The model under review builds one solid part; all positions refer to its coordinate system, in mm. Face numbers are marked on the shaded views. A direction names the side the tool comes from. Coordinates: 2 decimals unless noted, no trailing zeros. Order: outer loops, then holes, each group sorted by start corner. A loop starts at its lowest first (then second) coordinate and runs counter-clockwise, first axis right, second up.
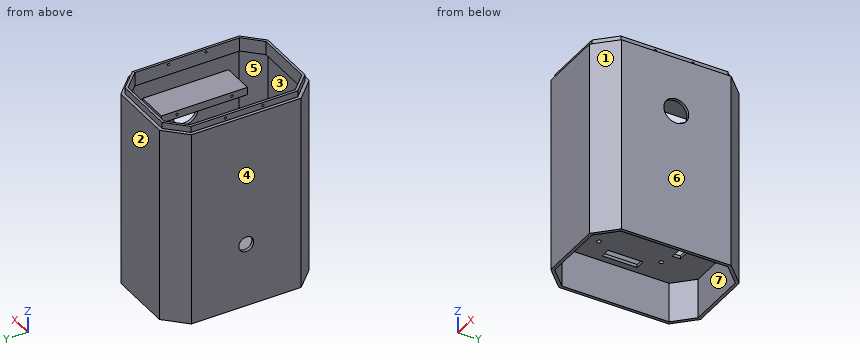
```python
from build123d import *

# Parameters (mm, degrees)
BOSS_1_DEPTH   = 157
CUT_2_DEPTH    = 122.675
CUT_3_DEPTH    = 32.025
S_CUT4_W       = 8
S_CUT4_H       = 28
POCKET_4_DEPTH = 2.7
S_HOLE5_R      = 6
HOLE_5_DEPTH   = 2.7
S_CUT6_W       = 19.4
S_CUT6_H       = 6.3
POCKET_6_DEPTH = 2.7
S_CUT7_W       = 19.4
S_CUT7_H       = 6.3
POCKET_7_DEPTH = 2.7
S_HOLE8_R      = 1.7
HOLE_8_DEPTH   = 2.7
S_HOLE9_R      = 1.7
HOLE_9_DEPTH   = 2.7
S_HOLE10_R     = 1.7
HOLE_10_DEPTH  = 2.7
S_HOLE11_R     = 1.7
HOLE_11_DEPTH  = 2.7
BOSS_12_DEPTH  = 6
BOSS_13_DEPTH  = 5.1
S_CYL14_R      = 3.2
BOSS_14_DEPTH  = 6.5
S_CYL15_R      = 3.2
BOSS_15_DEPTH  = 6.5
S_CYL16_R      = 3.2
BOSS_16_DEPTH  = 6.5
S_CYL17_R      = 3.2
BOSS_17_DEPTH  = 6.5
S_BOX18_W      = 25.8
S_BOX18_H      = 27.5
BOSS_18_DEPTH  = 6
S_BOX19_W      = 25.8
S_BOX19_H      = 27.5
BOSS_19_DEPTH  = 6
S_BOX20_W      = 25.8
S_BOX20_H      = 69
BOSS_20_DEPTH  = 6
CUT_21_DEPTH   = 11.2
S_HOLE22_R     = 0.9
HOLE_22_DEPTH  = 2.7
S_HOLE23_R     = 0.9
HOLE_23_DEPTH  = 2.7
S_HOLE24_R     = 0.9
HOLE_24_DEPTH  = 2.7
S_HOLE25_R     = 0.9
HOLE_25_DEPTH  = 2.7
S_HOLE26_R     = 0.9
HOLE_26_DEPTH  = 7.2
S_HOLE27_R     = 0.9
HOLE_27_DEPTH  = 7.2
S_HOLE28_R     = 0.9
HOLE_28_DEPTH  = 7.2
S_HOLE29_R     = 0.9
HOLE_29_DEPTH  = 7.2
S_HOLE30_R     = 10
HOLE_30_DEPTH  = 3.1
S_HOLE31_R     = 0.9
HOLE_31_DEPTH  = 9.1
S_HOLE32_R     = 0.9
HOLE_32_DEPTH  = 9.1
S_HOLE33_R     = 0.9
HOLE_33_DEPTH  = 9.1
S_HOLE34_R     = 0.9
HOLE_34_DEPTH  = 9.1


with BuildPart() as part:
    # S_prism1 → Boss_1 (new body)
    with BuildSketch(Plane.XY.offset(37)):
        Polygon((42, -44), (42, 44), (26, 60), (-26, 60), (-42, 44), (-42, -44), (-26, -60), (26, -60), align=None)
    extrude(amount=BOSS_1_DEPTH)

    # S_pcut2 → Cut_2 (cut)
    with BuildSketch(Plane.XY.offset(71.425)):
        Polygon((39.5, -42.964466094), (39.5, 42.964466094), (24.964466094, 57.5), (-24.964466094, 57.5), (-39.5, 42.964466094), (-39.5, -42.964466094), (-24.964466094, -57.5), (24.964466094, -57.5), align=None)
    extrude(amount=CUT_2_DEPTH, mode=Mode.SUBTRACT)

    # S_pcut3 → Cut_3 (cut)
    with BuildSketch(Plane.XY.offset(36.9)):
        Polygon((39.5, -42.964466094), (39.5, 42.964466094), (24.964466094, 57.5), (-24.964466094, 57.5), (-39.5, 42.964466094), (-39.5, -42.964466094), (-24.964466094, -57.5), (24.964466094, -57.5), align=None)
    extrude(amount=CUT_3_DEPTH, mode=Mode.SUBTRACT)

    # S_cut4 → Pocket_4 (cut)
    with BuildSketch(Plane.XY.offset(68.825)):
        with Locations((-30, 0)):
            Rectangle(S_CUT4_W, S_CUT4_H)
    extrude(amount=POCKET_4_DEPTH, mode=Mode.SUBTRACT)

    # S_hole5 → Hole_5 (cut)
    with BuildSketch(Plane(origin=(-42.1, 0, 0), x_dir=(0, 0, -1), z_dir=(1, 0, 0))):
        with Locations((-88, 0)):
            Circle(S_HOLE5_R)
    extrude(amount=HOLE_5_DEPTH, mode=Mode.SUBTRACT)

    # S_cut6 → Pocket_6 (cut)
    with BuildSketch(Plane.XY.offset(68.825)):
        with Locations((0, 30.95)):
            Rectangle(S_CUT6_W, S_CUT6_H)
    extrude(amount=POCKET_6_DEPTH, mode=Mode.SUBTRACT)

    # S_cut7 → Pocket_7 (cut)
    with BuildSketch(Plane.XY.offset(68.825)):
        with Locations((0, -30.95)):
            Rectangle(S_CUT7_W, S_CUT7_H)
    extrude(amount=POCKET_7_DEPTH, mode=Mode.SUBTRACT)

    # S_hole8 → Hole_8 (cut)
    with BuildSketch(Plane.XY.offset(68.825)):
        with Locations((-20, -25)):
            Circle(S_HOLE8_R)
    extrude(amount=HOLE_8_DEPTH, mode=Mode.SUBTRACT)

    # S_hole9 → Hole_9 (cut)
    with BuildSketch(Plane.XY.offset(68.825)):
        with Locations((-20, 25)):
            Circle(S_HOLE9_R)
    extrude(amount=HOLE_9_DEPTH, mode=Mode.SUBTRACT)

    # S_hole10 → Hole_10 (cut)
    with BuildSketch(Plane.XY.offset(68.825)):
        with Locations((24, -25)):
            Circle(S_HOLE10_R)
    extrude(amount=HOLE_10_DEPTH, mode=Mode.SUBTRACT)

    # S_hole11 → Hole_11 (cut)
    with BuildSketch(Plane.XY.offset(68.825)):
        with Locations((24, 25)):
            Circle(S_HOLE11_R)
    extrude(amount=HOLE_11_DEPTH, mode=Mode.SUBTRACT)

    # S_prism12 → Boss_12 (add)
    with BuildSketch(Plane.XY.offset(188)):
        Polygon((40, -43.171572875), (40, 43.171572875), (25.171572875, 58), (-25.171572875, 58), (-40, 43.171572875), (-40, -43.171572875), (-25.171572875, -58), (25.171572875, -58), align=None)
    extrude(amount=BOSS_12_DEPTH)

    # S_prism13 → Boss_13 (add)
    with BuildSketch(Plane.XY.offset(193.9)):
        Polygon((39.3, -42.881623382), (39.3, 42.881623382), (24.881623382, 57.3), (-24.881623382, 57.3), (-39.3, 42.881623382), (-39.3, -42.881623382), (-24.881623382, -57.3), (24.881623382, -57.3), align=None)
    extrude(amount=BOSS_13_DEPTH)

    # S_cyl14 → Boss_14 (add)
    with BuildSketch(Plane(origin=(-40, 0, 0), x_dir=(0, 0, -1), z_dir=(1, 0, 0))):
        with Locations((-96, -29)):
            Circle(S_CYL14_R)
    extrude(amount=BOSS_14_DEPTH)

    # S_cyl15 → Boss_15 (add)
    with BuildSketch(Plane(origin=(-40, 0, 0), x_dir=(0, 0, -1), z_dir=(1, 0, 0))):
        with Locations((-145, -29)):
            Circle(S_CYL15_R)
    extrude(amount=BOSS_15_DEPTH)

    # S_cyl16 → Boss_16 (add)
    with BuildSketch(Plane(origin=(-40, 0, 0), x_dir=(0, 0, -1), z_dir=(1, 0, 0))):
        with Locations((-96, 29)):
            Circle(S_CYL16_R)
    extrude(amount=BOSS_16_DEPTH)

    # S_cyl17 → Boss_17 (add)
    with BuildSketch(Plane(origin=(-40, 0, 0), x_dir=(0, 0, -1), z_dir=(1, 0, 0))):
        with Locations((-145, 29)):
            Circle(S_CYL17_R)
    extrude(amount=BOSS_17_DEPTH)

    # S_box18 → Boss_18 (add)
    with BuildSketch(Plane.XY.offset(126.2)):
        with Locations((27.1, -20.75)):
            Rectangle(S_BOX18_W, S_BOX18_H)
    extrude(amount=BOSS_18_DEPTH)

    # S_box19 → Boss_19 (add)
    with BuildSketch(Plane.XY.offset(126.2)):
        with Locations((27.1, 20.75)):
            Rectangle(S_BOX19_W, S_BOX19_H)
    extrude(amount=BOSS_19_DEPTH)

    # S_box20 → Boss_20 (add)
    with BuildSketch(Plane.XY.offset(167.8)):
        with Locations((27.1, 0)):
            Rectangle(S_BOX20_W, S_BOX20_H)
    extrude(amount=BOSS_20_DEPTH)

    # S_pcut21 → Cut_21 (cut)
    with BuildSketch(Plane.XY.offset(187.9)):
        Polygon((37.3, -42.053196257), (37.3, 42.053196257), (24.053196257, 55.3), (-24.053196257, 55.3), (-37.3, 42.053196257), (-37.3, -42.053196257), (-24.053196257, -55.3), (24.053196257, -55.3), align=None)
    extrude(amount=CUT_21_DEPTH, mode=Mode.SUBTRACT)

    # S_hole22 → Hole_22 (cut)
    with BuildSketch(Plane(origin=(37.1, 0, 0), x_dir=(0, 0, -1), z_dir=(1, 0, 0))):
        with Locations(Location((-196.5, -15, 0), (0, 0, 180))):
            Circle(S_HOLE22_R)
    extrude(amount=HOLE_22_DEPTH, mode=Mode.SUBTRACT)

    # S_hole23 → Hole_23 (cut)
    with BuildSketch(Plane(origin=(37.1, 0, 0), x_dir=(0, 0, -1), z_dir=(1, 0, 0))):
        with Locations(Location((-196.5, 15, 0), (0, 0, 180))):
            Circle(S_HOLE23_R)
    extrude(amount=HOLE_23_DEPTH, mode=Mode.SUBTRACT)

    # S_hole24 → Hole_24 (cut)
    with BuildSketch(Plane(origin=(-39.8, 0, 0), x_dir=(0, 0, -1), z_dir=(1, 0, 0))):
        with Locations(Location((-196.5, -15, 0), (0, 0, 180))):
            Circle(S_HOLE24_R)
    extrude(amount=HOLE_24_DEPTH, mode=Mode.SUBTRACT)

    # S_hole25 → Hole_25 (cut)
    with BuildSketch(Plane(origin=(-39.8, 0, 0), x_dir=(0, 0, -1), z_dir=(1, 0, 0))):
        with Locations(Location((-196.5, 15, 0), (0, 0, 180))):
            Circle(S_HOLE25_R)
    extrude(amount=HOLE_25_DEPTH, mode=Mode.SUBTRACT)

    # S_hole26 → Hole_26 (cut)
    with BuildSketch(Plane(origin=(-40.6, 0, 0), x_dir=(0, 0, -1), z_dir=(1, 0, 0))):
        with Locations((-96, -29)):
            Circle(S_HOLE26_R)
    extrude(amount=HOLE_26_DEPTH, mode=Mode.SUBTRACT)

    # S_hole27 → Hole_27 (cut)
    with BuildSketch(Plane(origin=(-40.6, 0, 0), x_dir=(0, 0, -1), z_dir=(1, 0, 0))):
        with Locations((-145, -29)):
            Circle(S_HOLE27_R)
    extrude(amount=HOLE_27_DEPTH, mode=Mode.SUBTRACT)

    # S_hole28 → Hole_28 (cut)
    with BuildSketch(Plane(origin=(-40.6, 0, 0), x_dir=(0, 0, -1), z_dir=(1, 0, 0))):
        with Locations((-96, 29)):
            Circle(S_HOLE28_R)
    extrude(amount=HOLE_28_DEPTH, mode=Mode.SUBTRACT)

    # S_hole29 → Hole_29 (cut)
    with BuildSketch(Plane(origin=(-40.6, 0, 0), x_dir=(0, 0, -1), z_dir=(1, 0, 0))):
        with Locations((-145, 29)):
            Circle(S_HOLE29_R)
    extrude(amount=HOLE_29_DEPTH, mode=Mode.SUBTRACT)

    # S_hole30 → Hole_30 (cut)
    with BuildSketch(Plane(origin=(39, 0, 0), x_dir=(0, 0, -1), z_dir=(1, 0, 0))):
        with Locations(Location((-150, 0, 0), (0, 0, 180))):
            Circle(S_HOLE30_R)
    extrude(amount=HOLE_30_DEPTH, mode=Mode.SUBTRACT)

    # S_hole31 → Hole_31 (cut)
    with BuildSketch(Plane(origin=(14.1, 0, 0), x_dir=(0, 0, -1), z_dir=(1, 0, 0))):
        with Locations((-129.2, -22)):
            Circle(S_HOLE31_R)
    extrude(amount=HOLE_31_DEPTH, mode=Mode.SUBTRACT)

    # S_hole32 → Hole_32 (cut)
    with BuildSketch(Plane(origin=(14.1, 0, 0), x_dir=(0, 0, -1), z_dir=(1, 0, 0))):
        with Locations((-170.8, -22)):
            Circle(S_HOLE32_R)
    extrude(amount=HOLE_32_DEPTH, mode=Mode.SUBTRACT)

    # S_hole33 → Hole_33 (cut)
    with BuildSketch(Plane(origin=(14.1, 0, 0), x_dir=(0, 0, -1), z_dir=(1, 0, 0))):
        with Locations((-129.2, 22)):
            Circle(S_HOLE33_R)
    extrude(amount=HOLE_33_DEPTH, mode=Mode.SUBTRACT)

    # S_hole34 → Hole_34 (cut)
    with BuildSketch(Plane(origin=(14.1, 0, 0), x_dir=(0, 0, -1), z_dir=(1, 0, 0))):
        with Locations((-170.8, 22)):
            Circle(S_HOLE34_R)
    extrude(amount=HOLE_34_DEPTH, mode=Mode.SUBTRACT)


solid = part.part
```
(1) Wall thickness on probe 1 along Z at (x, y) = (26.5, -15.5) (3 decimals); probe 2 along Y at (x, z) = (16.5, 129.2); probe 3 along X at (y, z) = (17.5, 117.5): over which ranges is each line inside the solid? List them lowest first.
A:
probe 1: z = 68.925 to 71.425, 126.2 to 132.2, 167.8 to 173.8
probe 2: y = -60 to -57.5, -34.5 to -22.9, -21.1 to -7, 7 to 21.1, 22.9 to 34.5, 57.5 to 60
probe 3: x = -42 to -39.5, 39.5 to 42
(2) Draft analysis for pull direction X (two halves, no side actions). For the marked faces 1, 2, 3 and 4, state which applies: released by +X, released by -X, zero draft, split by the parting line, or undercut.
A:
face 1: released by +X
face 2: zero draft
face 3: undercut
face 4: released by -X
(3) We need section B-B, the plane z = 136.5. Write out the cut boundary in (x, y), and give its area (3 significant figures).
A:
outline: (-42, -44) - (-26, -60) - (26, -60) - (42, -44) - (42, 44) - (26, 60) - (-26, 60) - (-42, 44) - close; hole (-39.5, -42.96) - (-24.96, -57.5) - (24.96, -57.5) - (39.5, -42.96) - (39.5, 42.96) - (24.96, 57.5) - (-24.96, 57.5) - (-39.5, 42.96) - close
area: 906 mm2
(4) We need section C-C, the plane y = 37. Write out the cut boundary in (x, z) (3 decimals), and give its area (3 significant figures).
A:
outline: (-42, 37) - (-39.5, 37) - (-39.5, 68.925) - (39.5, 68.925) - (39.5, 37) - (42, 37) - (42, 194) - (39.3, 194) - (39.3, 199) - (37.3, 199) - (37.3, 188) - (39.5, 188) - (39.5, 71.425) - (-39.5, 71.425) - (-39.5, 188) - (-37.3, 188) - (-37.3, 199) - (-39.3, 199) - (-39.3, 194) - (-42, 194) - close
area: 1,030 mm2
(5) Machinability: for the marked faces 5, 6 and 7, which of the approach directions +Z, -Z, +X, -X, +Y, -Y give a long, thin tool a straight path to every point of the face, cutting with its end or side? Answer none if there is none.
A:
face 5: none
face 6: +Z, -Z, +X, +Y, -Y
face 7: -Z
(6) We need section D-D, the plane x = -30. Write out the cut boundary in (y, z) (3 decimals).
A:
outline: (-56, 37) - (-52.464, 37) - (-52.464, 68.925) - (-14, 68.925) - (-14, 71.425) - (-52.464, 71.425) - (-52.464, 188) - (-49.353, 188) - (-49.353, 199) - (-52.182, 199) - (-52.182, 194) - (-56, 194) - close; (14, 68.925) - (52.464, 68.925) - (52.464, 37) - (56, 37) - (56, 194) - (52.182, 194) - (52.182, 199) - (49.353, 199) - (49.353, 188) - (52.464, 188) - (52.464, 71.425) - (14, 71.425) - close
(7) For pin 1 Ø2.5 at (x, z) = (-10, 196) entering from +Y; pin 2 Ø3 at (x, y) = (24.5, 17.5) entering from +Z; pin 3 Ø1 at (x, z) = (31, 109) entering from +Y; pin 4 Ø5.5 at (y, z) = (-18.5, 195.5) entering from +X, all flat-tipped, find the tip position at first contact; note any pin that passes through.
A:
pin 1: stops at y = 57.3
pin 2: stops at z = 173.8
pin 3: stops at y = 55.5
pin 4: stops at x = 42
